Autodesk Inventor part; units mm, degrees
ref_plane "YZ Plane" through (0, 0, 0) normal (1, 0, 0) x (0, 1, 0)
ref_plane "XZ Plane" through (0, 0, 0) normal (0, 1, 0) x (-1, 0, 0)
ref_plane "XY Plane" through (0, 0, 0) normal (0, 0, 1) x (1, 0, 0)
sketch "Эскиз1" plane through (0, 0, 0) normal (0, 0, 1) x (1, 0, 0)
  line L0 (-78.0042, 6) -> (-78.0042, 20)
  line L1 (-78.0042, 20) -> (-42.5, 20)
  line L2 (-32.5, 20) -> (-32.5, 17)
  line L3 (-32.5, 17) -> (-42.5, 17)
  line L4 (-42.5, 17) -> (-42.5, 20)
  line L5 (-32.5, 20) -> (-5, 20)
  line L6 (0, 17) -> (-5, 17)
  line L7 (-5, 17) -> (-5, 20)
  line L8 (-75.0118, -6.0217) -> (-75.0118, 6)
  line L9 (-75.0118, 6) -> (-78.0042, 6)
  line L10 (-78.0042, 20) -> (-42.5, 20)
  line L11 (-32.5, 20) -> (-5, 20)
  line L12 (77.9946, 6.1624) -> (77.9946, 20)
  line L13 (77.9946, 20) -> (42.5, 20)
  line L14 (32.5, 20) -> (32.5, 17)
  line L15 (32.5, 17) -> (42.5, 17)
  line L16 (42.5, 17) -> (42.5, 20)
  line L17 (32.5, 20) -> (5, 20)
  line L18 (0, 17) -> (5, 17)
  line L19 (5, 17) -> (5, 20)
  line L20 (74.9946, 0.1624) -> (74.9946, 6.1624)
  line L21 (74.9946, 6.1624) -> (77.9946, 6.1624)
  line L22 (77.9946, 20) -> (42.5, 20)
  line L23 (32.5, 20) -> (5, 20)
  line L24 (-78.0038, -6.0216) -> (-78.0038, -20)
  line L25 (-78.0038, -20) -> (-42.5, -20)
  line L26 (-32.5, -20) -> (-32.5, -17)
  line L27 (-32.5, -17) -> (-42.5, -17)
  line L28 (-42.5, -17) -> (-42.5, -20)
  line L29 (-32.5, -20) -> (-5, -20)
  line L30 (0, -17) -> (-5, -17)
  line L31 (-5, -17) -> (-5, -20)
  line L32 (-75.0118, -6.0217) -> (-75.0118, -6.0216)
  line L33 (-75.0118, -6.0216) -> (-78.0038, -6.0216)
  line L34 (-78.0038, -20) -> (-42.5, -20)
  line L35 (-32.5, -20) -> (-5, -20)
  line L36 (77.9946, -5.8376) -> (77.9946, -20)
  line L37 (77.9946, -20) -> (42.5, -20)
  line L38 (32.5, -20) -> (32.5, -17)
  line L39 (32.5, -17) -> (42.5, -17)
  line L40 (42.5, -17) -> (42.5, -20)
  line L41 (32.5, -20) -> (5, -20)
  line L42 (0, -17) -> (5, -17)
  line L43 (5, -17) -> (5, -20)
  line L44 (74.9946, 0.1624) -> (74.9946, -5.8376)
  line L45 (74.9946, -5.8376) -> (77.9946, -5.8376)
  line L46 (77.9946, -20) -> (42.5, -20)
  line L47 (32.5, -20) -> (5, -20)
  line L48 (-78.0042, 6) -> (-75.0042, 6)
  point P0 (0, 0)
extrude "Выдавливание1" add sketch "Эскиз1" along normal blind 3
properties part number "Стекнка t1"
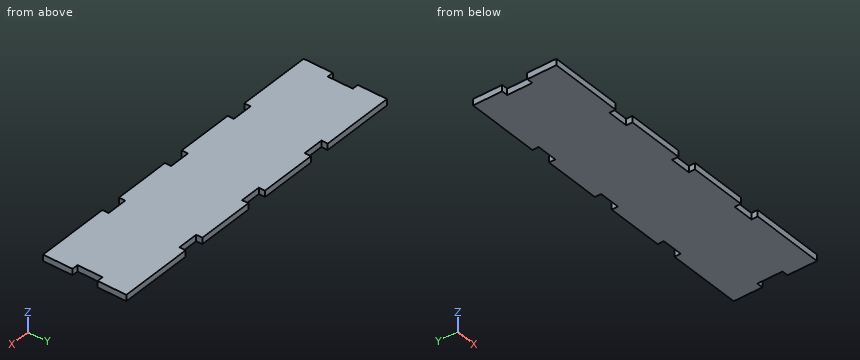
For this review, take the finished solid that the model builds, in its own axes (mm). Give positions to 0.01 mm unless a question says otherwise; leave off trailing zeros. Write each loop counter-clockwise with the first axis right and the second up, starting at its lowest first coordinate (ties: lowest second). Pieces come first, ordered by that corner, then holes. Notation, with made-up numbers: M 11.5,-27.5 L 50.5,-27.5 A25 cw 50.5,-13.5 Z; hole C -11.5,-17.75 d5. An arc over 180 degrees is marked long. Answer as a JSON object with one key per item and string values. Group by question number.
Item 1: Consider section A-A on y = 0. Write out the cut boundary in (x, z), plus the area to 3 significant figures.
Item 2: For probe 1 along X at (y, z) = (18, 1.55); probe 2 along X at (y, z) = (4, 1.05); probe 3 along Y at (x, z) = (40, 1.5), list the stretches that pass through material, from the lowest coordinate up. Write a range as [from, to].
Item 3: For pin 1 Ø1.5 at (x, z) = (36.5, 1.5) entering from +Y; pin 2 Ø0.9 at (y, z) = (2.5, 2) entering from +X; pin 3 Ø1.5 at (y, z) = (-1.5, 2) entering from -X, all flat-tipped, find the tip position at first contact; note any pin that passes through.
Check result:
{
 "1": {"outline": "M -75.01,0 L 74.99,0 L 74.99,3 L -75.01,3 Z", "area": "450 mm^2"},
 "2": {"probe 1": "x = [-78, -42.5], [-32.5, -5], [5, 32.5], [42.5, 77.99]", "probe 2": "x = [-75.01, 74.99]", "probe 3": "y = [-17, 17]"},
 "3": {"pin 1": "stops at y = 17", "pin 2": "stops at x = 74.99", "pin 3": "stops at x = -75.01"}
}
